from build123d import *

# Parameters (mm, degrees)
SKETCH1_R           = 2.5
BOSS_EXTRUDE1_DEPTH = 100
CUT_EXTRUDE1_DEPTH  = 2.5
BOSS_EXTRUDE2_DEPTH = 1
CHAMFER1_SIZE       = 1
CUT_EXTRUDE2_DEPTH  = 2.5
CUT_EXTRUDE3_DEPTH  = 2.5


with BuildPart() as part:
    # Sketch1 → Boss-Extrude1 (new body)
    with BuildSketch(Plane.XY):
        Circle(SKETCH1_R)
    extrude(amount=BOSS_EXTRUDE1_DEPTH)

    # Sketch2 → Cut-Extrude1 (cut, symmetric)
    with BuildSketch(Plane(origin=(0, 0, 0), x_dir=(0, 0, -1), z_dir=(1, 0, 0))):
        with BuildLine():
            Line((-94, 4), (-88, 4))
            ThreePointArc((-88, 4), (-87.292893219, 3.707106781), (-87, 3))
            Line((-87, 3), (-87, 2))
            ThreePointArc((-87, 2), (-87.292893219, 1.292893219), (-88, 1))
            Line((-88, 1), (-94, 1))
            ThreePointArc((-94, 1), (-94.707106781, 1.292893219), (-95, 2))
            Line((-95, 2), (-95, 3))
            ThreePointArc((-95, 3), (-94.707106781, 3.707106781), (-94, 4))
        make_face()
        with BuildLine():
            Line((-95, -3), (-95, -2))
            ThreePointArc((-95, -2), (-94.707106781, -1.292893219), (-94, -1))
            Line((-94, -1), (-88, -1))
            ThreePointArc((-88, -1), (-87.292893219, -1.292893219), (-87, -2))
            Line((-87, -2), (-87, -3))
            ThreePointArc((-87, -3), (-87.292893219, -3.707106781), (-88, -4))
            Line((-88, -4), (-94, -4))
            ThreePointArc((-94, -4), (-94.707106781, -3.707106781), (-95, -3))
        make_face()
    extrude(amount=CUT_EXTRUDE1_DEPTH, both=True, mode=Mode.SUBTRACT)

    # Sketch2<2> → Boss-Extrude2 (add, symmetric)
    with BuildSketch(Plane(origin=(0, 0, 0), x_dir=(0, 0, -1), z_dir=(1, 0, 0))):
        with BuildLine():
            Line((-94, 4), (-88, 4))
            ThreePointArc((-88, 4), (-87.292893219, 3.707106781), (-87, 3))
            Line((-87, 3), (-87, 2))
            ThreePointArc((-87, 2), (-87.292893219, 1.292893219), (-88, 1))
            Line((-88, 1), (-94, 1))
            ThreePointArc((-94, 1), (-94.707106781, 1.292893219), (-95, 2))
            Line((-95, 2), (-95, 3))
            ThreePointArc((-95, 3), (-94.707106781, 3.707106781), (-94, 4))
        make_face()
        with BuildLine():
            Line((-95, -3), (-95, -2))
            ThreePointArc((-95, -2), (-94.707106781, -1.292893219), (-94, -1))
            Line((-94, -1), (-88, -1))
            ThreePointArc((-88, -1), (-87.292893219, -1.292893219), (-87, -2))
            Line((-87, -2), (-87, -3))
            ThreePointArc((-87, -3), (-87.292893219, -3.707106781), (-88, -4))
            Line((-88, -4), (-94, -4))
            ThreePointArc((-94, -4), (-94.707106781, -3.707106781), (-95, -3))
        make_face()
    extrude(amount=BOSS_EXTRUDE2_DEPTH, both=True)

    # Chamfer1
    chamfer1_edges = [part.edges().sort_by_distance(p)[0] for p in [
        (-2.5, 0, 100),
    ]]
    chamfer(chamfer1_edges, length=CHAMFER1_SIZE)

    # Sketch3 → Cut-Extrude2 (cut, symmetric)
    with BuildSketch(Plane(origin=(0, 0, 0), x_dir=(0, 0, -1), z_dir=(1, 0, 0))):
        Polygon((0, -2.5), (0, 0), (-15, -2.5), align=None)
        Polygon((-15, 2.5), (0, 0), (0, 2.5), align=None)
    extrude(amount=CUT_EXTRUDE2_DEPTH, both=True, mode=Mode.SUBTRACT)

    # Sketch4 → Cut-Extrude3 (cut, symmetric)
    with BuildSketch(Plane(origin=(0, 0, 0), x_dir=(1, 0, 0), z_dir=(0, 1, 0))):
        Polygon((-2.5, -15), (0, 0), (-2.5, 0), align=None)
        Polygon((2.5, 0), (0, 0), (2.5, -15), align=None)
    extrude(amount=CUT_EXTRUDE3_DEPTH, both=True, mode=Mode.SUBTRACT)


solid = part.part
Model file for the job. Use its own axes, mm. A direction names the side the tool comes from. Give positions to 0.01 mm unless a question says otherwise; leave off trailing zeros. Write each loop counter-clockwise with the first axis right and the second up, starting at its lowest first coordinate (ties: lowest second). Pieces come first, ordered by that corner, then holes. Notation, with made-up numbers: (-1, 23.5) - (26, 23.5) arc R19 cw to (26, 28.5) - close; hole circle Ø11 at (85, 87). An arc over 180 degrees is marked (long way). Answer as CSV lines item,"result".
1. 3-axis set-ups, long thin cutter, end or side, ignore diameter. For faces 1 (the face through (-1, 3, 91)), 2 (the face through (-1, -2, 91)), 3 (the face through (0.025, 1.545, 9.272)), 4 (the face through (1, 3, 91)): which of +Z, -Z, +X, -X, +Y, -Y reach the whole face in a straight line?
Responses:
face 1,"-X, +Y"
face 2,"-X, -Y"
face 3,"-Z, +X, -X, +Y"
face 4,"+X, +Y"
2. Two-plate mould, pull along Z, no slides. Class faces 5 (the face through (0, 4, 91)), 6 (the face through (1, -2, 91)), 7 (the face through (0, 0, 100)), 8 (the face through (1.51, 0.02, 9.06)): +Z half, -Z half, draft (parallel to the pull), parting line (faces both ways), or undercut.
Responses:
face 5,"draft"
face 6,"undercut"
face 7,"+Z half"
face 8,"-Z half"
3. Band-saw the part on A-A (z = 12). Write the cut outline in (x, y).
Responses:
outline,"(-2, -1.5) arc R2.5 ccw to (-1.5, -2) - (1.5, -2) arc R2.5 ccw to (2, -1.5) - (2, 1.5) arc R2.5 ccw to (1.5, 2) - (-1.5, 2) arc R2.5 ccw to (-2, 1.5) - close"
4. Drill centre lines: L1, parallel to Y at x = -0.15, z = 59; L2, parallel to Y at x = 1.2, z = 91; L3, parallel to Z at x = -0.1, y = 3. Where is each one in solid material? Low to high. Write a range as [from, to].
Responses:
L1,"y = [-2.5, 2.5]"
L2,"y = [-1, 1]"
L3,"z = [87, 95]"
5. Band-saw the part on B-B (z = 51.5). Write the cut outline in (x, y).
Responses:
outline,"circle Ø5 at (0, 0)"
6. Pin check, flat tips, straight feed: pin 1 (2.5 mm diameter, centred on y = 2.5, z = 90.5, fed in from -X); pin 2 (1 mm diameter, centred on x = 0.5, y = 3, fed in from -Z); pin 3 (2 mm diameter, centred on x = 2, z = 14, fed in from -Y). Stop position of each tip, or through.
Responses:
pin 1,"stops at x = -1"
pin 2,"stops at z = 87"
pin 3,"stops at y = -2.29"
